Print and shaded views of the part. All mm, measured from the part's lowest x, y and z. Coordinates: 2 decimals unless noted, no trailing zeros. Order: outer loops, then holes, each group sorted by start corner. A loop starts at its lowest first (then second) coordinate and runs counter-clockwise, first axis right, second up.
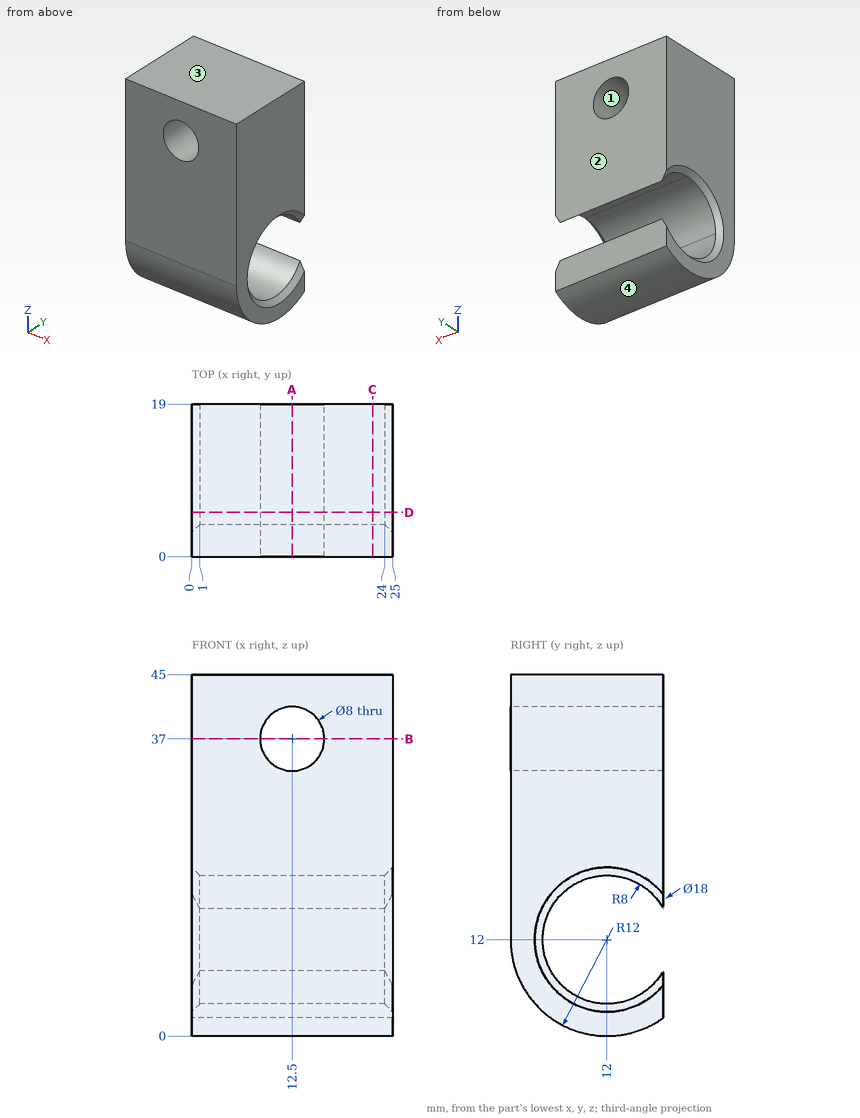
Q1. Probe line 1 (Z direction, x = 12.5, y = 6.25); line 2 (Z direction, x = 13.5, y = 11.5); line 3 (Z direction, x = 19, y = 10.25). List the from-to ranges inside material, lowest first.
Established:
line 1: z = 1.47 to 6.44, 17.56 to 33, 41 to 45
line 2: z = 0.01 to 4.02, 19.98 to 33.13, 40.87 to 45
line 3: z = 0.13 to 4.19, 19.81 to 45
Q2. Cut at B-B, the plane z = 37. List the corners of the cut face in (x, y), plus the area to 3 significant figures.
Established:
outline: (0, 0) - (8.5, 0) - (8.5, 19) - (0, 19) - close; (16.5, 0) - (25, 0) - (25, 19) - (16.5, 19) - close
area: 323 mm2
Q3. Cut at A-A, the plane x = 12.5. List the corners of the cut face in (y, z).
Established:
outline: (0, 12) arc R12 ccw to (19, 2.25) - (19, 8.13) arc R8 cw (long way) to (19, 15.87) - (19, 33) - (0, 33) - close; (0, 41) - (19, 41) - (19, 45) - (0, 45) - close
Q4. Cut at D-D, the plane y = 5.5. Count the separate pieces of the cut face and the enclosed holes in it, plus the area to 3 significant figures.
Established:
separate pieces: 2
enclosed holes: 1
area: 791 mm2
Q5. Cut at C-C, the plane x = 22.5. List the corners of the cut face in (y, z).
Established:
outline: (0, 12) arc R12 ccw to (19, 2.25) - (19, 8.13) arc R8 cw (long way) to (19, 15.87) - (19, 45) - (0, 45) - close
Q6. Mould opens along Z. For the marked faces 1, 2, 3 and 4 say: pulls with the +Z half, pulls with the -Z half, needs draft (parallel to the pull), parting line crosses it, or undercut.
Established:
face 1: undercut
face 2: needs draft
face 3: pulls with the +Z half
face 4: pulls with the -Z half
